Could you check a few things on this model? Use its own coordinates, in mm. A direction names the side the tool comes from. Give positions to 0.01 mm unless a question says otherwise; leave off trailing zeros. Write each loop counter-clockwise with the first axis right and the second up, starting at its lowest first coordinate (ties: lowest second). Pieces come first, ordered by that corner, then holes. Notation, with made-up numbers: (-23.5, 46) - (-16.5, 46) arc R25 cw to (-16.5, 74) - close; hole circle Ø7 at (71, 75). An arc over 180 degrees is marked (long way). Answer as CSV lines item,"result". Start each with the question number.
Q1. Imagine slicing it at B-B on z = -81.5. List the corners of the cut face in (x, y) for me (3 decimals).
Q2. Imagine slicing it at D-D on x = -18. List the corners of the cut face in (y, z) for me (3 decimals), and give its area (3 significant figures).
Q3. On a 3-axis mill with a long thin cutter (end or side, diameter ignored), from which of +Z, -Z, +X, -X, +Y, -Y can I reach the whole of each face in a straight line? I mean faces 4 (the face through (40.125, 0, -84)), 5 (the face through (-53, 24, -180)), 6 (the face through (35, 29.125, -162)). Say none if no direction works.
Q4. Imagine slicing it at A-A on x = 11. List the corners of the cut face in (y, z) for me (3 decimals), and give its area (3 significant figures).
Q5. Imagine slicing it at C-C on y = 2.5. List the corners of the cut face in (x, z) for me (3 decimals).
Q6. If I drill on line 1 along X through (y, z) = (-11.5, -64.5) (3 decimals); line 2 along Y through (x, z) = (-39, -46) (3 decimals); line 3 along X through (y, z) = (14.5, -156.5) (3 decimals), over which ranges is the centre line in solid material (lowest first)?
Q7. We'd pull the mould along Z, two halves only. Please class faces 1 (the face through (-52, 25, -187.5)), 2 (the face through (55, 23, -179)), 3 (the face through (44, -13.66, -70.83)): pulls with the +Z half, pulls with the -Z half, needs draft (parallel to the pull), parting line crosses it, or undercut.
Q8. Will these pins go through, and if not, where does the flat tip stop? pin 1 Ø1 at (x, y) = (-57.5, -15.5) entering from +Z; pin 2 Ø2.5 at (y, z) = (-14, -111) entering from -X; pin 3 Ø2.5 at (x, y) = (5, -13) entering from +Z; pin 4 Ø2 at (x, z) = (-44, -162.5) entering from +Y.
Autodesk Inventor part; units mm, degrees
ref_plane "作業平面6" through (53, 16.1124, -189.5) normal (0, 0, 1) x (1, 0, 0)
ref_plane "作業平面9" through (42.125, -17.075, 0) normal (0, 0, 1) x (0, 1, 0)
ref_plane "YZ Plane" through (0, 0, 0) normal (1, 0, 0) x (0, 1, 0)
sketch "スケッチ1" plane through (0, 0, 0) normal (0, 0, 1) x (1, 0, 0)
  line L0 (-42.125, -17.075) -> (42.125, -17.075)
  line L1 (42.125, -17.075) -> (42.125, 15.125)
  line L2 (42.125, 15.125) -> (-42.125, 15.125)
  line L3 (-42.125, 15.125) -> (-42.125, -17.075)
  point P0 (0, 0)
  dimension "d0" = 84.25
  dimension "d1" = 32.2
  dimension "d140" = 15.125
extrude "本体＿側" add sketch "スケッチ1" against normal blind 174
sketch "スケッチ3" plane through (0, 0, 0) normal (0, 0, 1) x (1, 0, 0)
  line L0 (-40.125, -12.075) -> (40.125, -12.075)
  line L1 (40.125, -12.075) -> (40.125, 13.125)
  line L2 (40.125, 13.125) -> (-40.125, 13.125)
  line L3 (-40.125, 13.125) -> (-40.125, -12.075)
  line L4 (42.125, 15.125) -> (-42.125, 15.125)
  line L5 (-42.125, -17.075) -> (42.125, -17.075)
  line L6 (-42.125, 15.125) -> (-42.125, -17.075)
  dimension "d4" = 80.25
  dimension "d125" = 2
  dimension "d138" = 2
  dimension "d139" = 25.2
extrude "本体" cut sketch "スケッチ3" against normal blind 170
sketch "スケッチ6" plane through (0, 0, -174) normal (0, 0, -1) x (-1, 0, 0)
  line L0 (55, 48.1251) -> (-55, 48.1251)
  line L1 (-55, 48.1251) -> (-55, 14.1251)
  line L2 (-55, 14.1251) -> (55, 14.1251)
  line L3 (55, 14.1251) -> (55, 48.1251)
  line L4 (55, 48.1251) -> (-55, 14.1251) construction
  line L5 (-55, 48.1251) -> (55, 14.1251) construction
  line L6 (0, 0) -> (0, 97.4837)
  point P0 (0, 31.1251)
  point P1 (0, 31.1251)
  dimension "d8" = 110
  dimension "d9" = 34
extrude "カメラ" add sketch "スケッチ6" along normal blind 15.5 and the other way blind 4.5
sketch "スケッチ7" plane through (0, 0, -189.5) normal (0, 0, -1) x (-1, 0, 0)
  line L0 (-55, 48.1251) -> (-55, 14.1251)
  line L1 (-53, 16.1124) -> (53, 16.1124)
  line L2 (53, 16.1124) -> (53, 46.2624)
  line L3 (53, 46.2624) -> (-53, 46.2624)
  line L4 (-53, 46.2624) -> (-53, 16.1124)
  line L5 (-53, 16.1124) -> (53, 46.2624) construction
  line L6 (53, 16.1124) -> (-53, 46.2624) construction
  point P0 (0, 0)
  point P1 (-55, 31.1251)
  point P2 (-55, 31.1251)
  point P3 (0, 31.1874)
  point P4 (0, 31.1874)
  dimension "d14" = 30.15
  dimension "d15" = 106
extrude "カメラ＿本体" cut sketch "スケッチ7" against normal blind 18
ref_plane "作業平面1" through (-55, 31.1251, -189.5) normal (0, 1, 0) x (1, 0, 0)
ref_plane "作業平面2" through (0, 14.1251, -189.5) normal (-1, 0, 0) x (0, 0, 1)
sketch "スケッチ10" plane through (-53, 16.1124, -189.5) normal (0, 1, 0) x (1, 0, 0)
  line L0 (59.8, -12.45) -> (46.2, -12.45)
  line L1 (46.2, -12.45) -> (46.2, 0)
  line L2 (46.2, 0) -> (59.8, 0)
  line L3 (59.8, 0) -> (59.8, -12.45)
  line L4 (59.8, -12.45) -> (46.2, 0) construction
  line L5 (46.2, -12.45) -> (59.8, 0) construction
  line L6 (108, -20) -> (-2, -20)
  line L7 (53, -20) -> (53, -4.9349)
  line L8 (53, -227.4) -> (53, 37.9)
  line L9 (0, 0) -> (106, 0)
  line L10 (0, 0) -> (106, 0)
  line L11 (0, 0) -> (0, -18)
  line L12 (0, -18) -> (106, -18)
  line L13 (106, 0) -> (106, -18)
  point P0 (53, -189.5)
  point P1 (53, -6.225)
  point P2 (53, 0)
  dimension "d22" = 12.45
  dimension "d23" = 13.6
sketch "スケッチ11" plane through (0, 0, -169.5) normal (0, 0, 1) x (1, 0, 0)
  line L0 (-15, 22.8501) -> (15, 22.8501)
  line L1 (15, 22.8501) -> (15, 39.4001)
  line L2 (15, 39.4001) -> (-15, 39.4001)
  line L3 (-15, 39.4001) -> (-15, 22.8501)
  line L4 (-53, 31.1251) -> (53, 31.1251)
  line L5 (-15, 22.8501) -> (15, 39.4001) construction
  line L6 (15, 22.8501) -> (-15, 39.4001) construction
  line L7 (0, -24.4525) -> (0, 47.8399)
  point P0 (0, 0)
  point P1 (0, 31.1251)
  point P2 (0, 31.1251)
  dimension "d26" = 30
  dimension "d27" = 16.55
extrude "突起" cut sketch "スケッチ10" against normal blind 2 contours L0 L7 L8 L2 L3 | L0 L1 L2 L8 L7
extrude "コード" cut sketch "スケッチ11" against normal blind 2
ref_plane "作業平面6" through (53, 16.1124, -189.5) normal (0, 0, 1) x (1, 0, 0)
sketch "スケッチ18" plane through (53, 16.1124, -189.5) normal (0, 0, 1) x (1, 0, 0)
  line L0 (0, 0) -> (0, 30.15)
  ellipse E0 centre (0, 15.0748) end of major axis (0, 0) minor radius 3.8117 (0, 30.1495) -> (0, 0) ccw
  line L1 (0, 30.15) -> (-106, 30.15)
  line L2 (-106, 0) -> (0, 0)
  line L3 (0, 30.15) -> (0, 0)
  point P0 (-53, -16.1124)
extrude "半円１" add sketch "スケッチ18" along normal blind 2
sketch "スケッチ19" plane through (53, 16.1124, -189.5) normal (0, 0, 1) x (1, 0, 0)
  line L0 (-106, 30.15) -> (-106, 0)
  ellipse E0 centre (-106.01, 15.0751) end of major axis (-106.0154, 30.1501) minor radius 3.8117 (-106.01, 0) -> (-106.01, 30.1501) ccw
  line L1 (-38, 6.7377) -> (-38, 23.2877)
  line L2 (-38, 23.2877) -> (-68, 23.2877)
  line L3 (-68, 23.2877) -> (-68, 6.7377)
  line L4 (-68, 6.7377) -> (-38, 6.7377)
  line L5 (-106, 0) -> (0, 0)
  line L6 (-106, 30.15) -> (-106, 0)
  line L7 (0, 30.15) -> (-106, 30.15)
  line L8 (0, 0) -> (0, 30.15)
  line L9 (-106, 0) -> (0, 0)
  line L10 (0, 30.15) -> (-106, 30.15)
  line L11 (-106, 0) -> (-106, 30.15)
  point P0 (-53, -16.1124)
extrude "半円2" add sketch "スケッチ19" along normal blind 2 contours E0 L0
sketch "スケッチ16" plane through (-55, 31.1251, -189.5) normal (0, 1, 0) x (1, 0, 0)
  line L0 (110, -20) -> (110, 0)
  line L1 (0, -20) -> (0, 0)
  line L2 (110, 0) -> (0, 0)
  line L3 (0, 0) -> (0, -20)
  line L4 (0, -20) -> (110, -20)
  line L5 (110, -20) -> (110, 0)
  point P0 (55, -189.5)
extrude "上半分消去" cut sketch "スケッチ16" along normal blind 17
sketch "スケッチ20" plane through (-42.125, 15.125, 0) normal (0, 1, 0) x (1, 0, 0)
  line L0 (18, 0) -> (66.25, 0)
  line L1 (66.25, 0) -> (66.25, 170)
  line L2 (66.25, 170) -> (18, 170)
  line L3 (18, 170) -> (18, 0)
  line L4 (18, 0) -> (66.25, 170) construction
  line L5 (66.25, 0) -> (18, 170) construction
  line L6 (84.25, 0) -> (0, 0)
  line L7 (42.125, -37.9) -> (42.125, 227.4)
  point P0 (42.125, 85)
  point P1 (42.125, 0)
  point P2 (42.125, 85)
  dimension "d47" = 170
  dimension "d91" = 18
extrude "ボタン部" cut sketch "スケッチ20" against normal blind 2
ref_plane "作業平面7" through (-42.125, 15.125, 0) normal (-1, 0, 0) x (0, 0, -1)
sketch "スケッチ22" plane through (-42.125, 15.125, 0) normal (-1, 0, 0) x (0, 0, -1)
  line L0 (0, 0) -> (174, 0)
  line L1 (169.5, 0) -> (154.5, 0)
  line L2 (154.5, 0) -> (154.5, -14)
  line L3 (154.5, -14) -> (169.5, -14)
  line L4 (169.5, -14) -> (169.5, 0)
  point P0 (0, 15.125)
  point P1 (169.5, 0.9999)
  dimension "d51" = 15
  dimension "d52" = 14
extrude "支え１" add sketch "スケッチ22" against normal blind 15
ref_plane "作業平面8" through (42.125, 15.125, 0) normal (-1, 0, 0) x (0, 0, -1)
sketch "スケッチ23" plane through (42.125, 15.125, 0) normal (-1, 0, 0) x (0, 0, -1)
  line L0 (0, 0) -> (174, 0)
  line L1 (154.5, -14) -> (154.5, 0)
  line L2 (169.5, 0) -> (154.5, 0)
  line L3 (154.5, 0) -> (154.5, -14)
  line L4 (154.5, -14) -> (169.5, -14)
  line L5 (169.5, -14) -> (169.5, 0)
  point P0 (0, 15.125)
  dimension "d55" = 15
  dimension "d56" = 14
extrude "支え２" add sketch "スケッチ23" along normal blind 15
ref_plane "作業平面9" through (42.125, -17.075, 0) normal (0, 0, 1) x (0, 1, 0)
sketch "スケッチ24" plane through (42.125, -17.075, 0) normal (0, 0, 1) x (0, 1, 0)
  line L0 (0, 84.25) -> (31.2001, 84.25)
  line L1 (0, 0) -> (0, 84.25)
  line L2 (28.25, 84.25) -> (0, 84.25)
  line L3 (0, 84.25) -> (0, 0)
  line L4 (0, 0) -> (28.25, 0)
  line L5 (28.25, 0) -> (28.25, 84.25)
  point P0 (17.075, 42.125)
extrude "削除予定" [suppressed]
sketch "スケッチ43" plane through (0, 0, 0) normal (0, 0, 1) x (1, 0, 0)
  line L0 (40.125, -12.075) -> (-40.125, -12.075)
  line L1 (0, -12.075) -> (31, -12.075)
  line L2 (26.4993, -15.075) -> (26.4993, -12.075)
  line L3 (26.4993, -12.075) -> (35.4993, -12.075)
  line L4 (35.4993, -12.075) -> (35.4993, -15.075)
  line L5 (35.4993, -15.075) -> (26.4993, -15.075)
  line L6 (26.4993, -15.075) -> (35.4993, -12.075) construction
  line L7 (26.4993, -12.075) -> (35.4993, -15.075) construction
  line L8 (30.9993, -12.075) -> (30.9993, -17.075)
  line L9 (-42.125, -17.075) -> (42.125, -17.075)
  point P0 (0, 0)
  point P1 (31, -12.125)
  dimension "d127" = 31
  dimension "d128" = 3
  dimension "d130" = 9
extrude "ネジ山溝１" cut sketch "スケッチ43" against normal blind 170
sketch "スケッチ44" plane through (0, 0, 0) normal (0, 0, 1) x (1, 0, 0)
  line L0 (26.4993, -12.075) -> (-40.125, -12.075)
  line L1 (0, -12.075) -> (-31, -12.075)
  line L2 (0, -30.115) -> (0, 61.1651)
  line L3 (-26.5, -15.075) -> (-26.5, -12.075)
  line L4 (-26.5, -12.075) -> (-35.5, -12.075)
  line L5 (-35.5, -12.075) -> (-35.5, -15.075)
  line L6 (-35.5, -15.075) -> (-26.5, -15.075)
  line L7 (-26.5, -15.075) -> (-35.5, -12.075) construction
  line L8 (-26.5, -12.075) -> (-35.5, -15.075) construction
  line L9 (-42.125, -17.075) -> (42.125, -17.075)
  line L10 (-31, -17.075) -> (-31, -12.075)
  point P0 (0, 0)
  point P1 (-31, -13.575)
  point P2 (-31, -13.575)
  dimension "d133" = 31
  dimension "d134" = 9
  dimension "d135" = 3
extrude "ネジ山溝２" cut sketch "スケッチ44" against normal blind 170 contours L3 L6 L10 L0 | L10 L6 L5 L0
sketch "スケッチ47" plane through (42.125, -17.075, 0) normal (1, 0, 0) x (0, 0, -1)
  line L0 (0, 0) -> (174, 0)
  line L1 (75, 2) -> (106, 2)
  line L2 (106, 2) -> (106, 0)
  line L3 (106, 0) -> (75, 0)
  line L4 (75, 0) -> (75, 2)
  line L5 (174, 31.2001) -> (174, 0)
  point P0 (0, 17.075)
  dimension "d141" = 68
  dimension "d142" = 31
  dimension "d145" = 2
extrude "押し出し28" add sketch "スケッチ47" along normal blind 31
sketch "スケッチ48" plane through (42.125, -15.075, -75) normal (0, 1, 0) x (1, 0, 0)
  point P0 (-42.125, -75)
fillet "フィレット1" radius 10 1 edges at (42.125, -15.075, -90.5)
fillet "フィレット2" radius 10 1 edges at (42.125, -16.075, -106)
fillet "フィレット3" radius 10 1 edges at (42.125, -16.075, -75)
sketch "スケッチ49" plane through (-42.125, -17.075, 0) normal (-1, 0, 0) x (0, 0, 1)
  line L0 (0, 0) -> (-174, 0)
  line L1 (-106, 0) -> (-75, 0)
  line L2 (-75, 0) -> (-75, 2)
  line L3 (-75, 2) -> (-106, 2)
  line L4 (-106, 2) -> (-106, 0)
  line L5 (-174, 0) -> (-174, 31.2001)
  point P0 (0, 17.075)
  dimension "d149" = 68
  dimension "d150" = 31
  dimension "d151" = 2
extrude "押し出し29" add sketch "スケッチ49" along normal blind 31
fillet "フィレット4" radius 10 1 edges at (-42.125, -15.075, -90.5)
fillet "フィレット5" radius 10 1 edges at (-42.125, -16.075, -75)
fillet "フィレット6" radius 10 1 edges at (-42.125, -16.075, -106)
sketch "スケッチ56" plane through (0, 0, 0) normal (0, 0, 1) x (1, 0, 0)
  line L0 (26.4993, -12.075) -> (-26.5, -12.075)
  line L1 (35.4993, -15.075) -> (26.4993, -15.075)
  line L2 (-26.5, -12.075) -> (26.4993, -12.075)
  line L3 (26.4993, -12.075) -> (26.4993, -15.075)
  line L4 (26.4993, -15.075) -> (-26.5, -15.075)
  line L5 (-26.5, -15.075) -> (-26.5, -12.075)
  point P0 (0, 0)
extrude "キャスターネジ溝" cut sketch "スケッチ56" against normal blind 35
properties part number "battery_case_1"
Conclusion:
1,outline,"(-73.125, -17.075) - (73.125, -17.075) - (73.125, -15.075) - (52.125, -15.075) arc R10 cw to (42.125, -5.075) - (42.125, 15.125) - (24.125, 15.125) - (24.125, 13.125) - (40.125, 13.125) - (40.125, -12.075) - (35.499, -12.075) - (35.499, -15.075) - (26.499, -15.075) - (26.499, -12.075) - (-26.5, -12.075) - (-26.5, -15.075) - (-35.5, -15.075) - (-35.5, -12.075) - (-40.125, -12.075) - (-40.125, 13.125) - (-24.125, 13.125) - (-24.125, 15.125) - (-42.125, 15.125) - (-42.125, -5.075) arc R10 cw to (-52.125, -15.075) - (-73.125, -15.075) - close"
2,outline,"(-17.075, -174) - (14.125, -174) - (14.125, -189.5) - (16.112, -189.5) - (16.112, -171.5) - (31.125, -171.5) - (31.125, -169.5) - (15.125, -169.5) - (15.125, -170) - (-12.075, -170) - (-12.075, -35) - (-15.075, -35) - (-15.075, 0) - (-17.075, 0) - close"
2,area,"939 mm^2"
3,face 4,"+Z"
3,face 5,"+Y"
3,face 6,"+Z, +X, -X, +Y"
4,outline,"(-17.075, -174) - (14.125, -174) - (14.125, -189.5) - (16.112, -189.5) - (16.112, -171.5) - (22.85, -171.5) - (22.85, -169.5) - (15.125, -169.5) - (15.125, -170) - (-12.075, -170) - (-12.075, -35) - (-15.075, -35) - (-15.075, 0) - (-17.075, 0) - close"
4,area,"923 mm^2"
5,outline,"(-42.125, -174) - (42.125, -174) - (42.125, 0) - (40.125, 0) - (40.125, -170) - (-40.125, -170) - (-40.125, 0) - (-42.125, 0) - close"
6,line 1,"-42.125 to -40.125, 40.125 to 42.125"
6,line 2,"-17.075 to -12.075, 13.125 to 15.125"
6,line 3,"-42.125 to -24.125, 24.125 to 42.125"
7,face 1,"undercut"
7,face 2,"needs draft"
7,face 3,"pulls with the +Z half"
8,pin 1,"z = -75"
8,pin 2,"x = -44.32"
8,pin 3,"z = -35"
8,pin 4,"through"
